Source: CAD feature listing. Evaluate the final solid. Frame: model axes, mm. Face numbers are marked on the shaded views. A direction names the side the tool comes from. Round coordinates to 2 decimals unless told otherwise and drop trailing zeros. Order: outer loops, then holes, each group sorted by start corner. A loop starts at its lowest first (then second) coordinate and runs counter-clockwise, first axis right, second up. Notation, with made-up numbers: M -12.75,17 L -6.75,17 A27 ccw -6.75,51 Z; hole C -12.5,73.25 d9. An arc over 180 degrees is marked long. Use one line per item in the form item = value. Start each with the question number.
Q1. Pull-direction query (X, two-part tool) for the marked faces 4, 5, 6 and 7; classes: pulls with the +X half, pulls with the -X half, needs draft (parallel to the pull), parting line crosses it, or undercut.
Q2. Section A-A (x = 13.5). Return the cut outline in (y, z), plus the area to 3 significant figures.
Q3. Section B-B (y = 2.3). Give the number of separate pieces and of enclosed holes in the cut face, plus the area to 3 significant figures.
Q4. Material intervals for probe 1 along X at (y, z) = (2.5, -6); probe 2 along Z at (x, y) = (52, 0.9); probe 3 along Z at (x, y) = (52, 1.15), sorted ascending.
Q5. Reachability of the marked faces 1, 2 and 3 from +Z, -Z, +X, -X, +Y, -Y: full face, straight path, thin tool, end or side. Return the list, or none.
Q6. Contact query for flat-ended pins moving along their axis: pin 1 (1.5 mm diameter, centred on x = 33.5, y = 4, fed in from -Z); pin 2 (1.5 mm diameter, centred on y = 2, z = -0.5, fed in from +X); pin 3 (3.5 mm diameter, centred on x = 0, z = 0, fed in from -Y); pin 4 (2.5 mm diameter, centred on x = 37, z = 0, fed in from -Y). Output: stop coordinate, or through.
from build123d import *

# Parameters (mm, degrees)
SKETCH1_W           = 10
SKETCH1_H           = 6
BOSS_EXTRUDE1_DEPTH = 5
BOSS_EXTRUDE3_DEPTH = 1
BOSS_EXTRUDE4_DEPTH = 7
SKETCH4_W           = 6
SKETCH4_H           = 5
BOSS_EXTRUDE5_DEPTH = 30
SKETCH5_W           = 14
SKETCH5_H           = 10
BOSS_EXTRUDE6_DEPTH = 5
FILLET17_R          = 5
SKETCH8_W           = 18
SKETCH8_H           = 5
BOSS_EXTRUDE7_DEPTH = 6
FILLET8_R           = 1
CUT_EXTRUDE3_DEPTH  = 15
SKETCH10_R          = 1.6
CUT_EXTRUDE4_DEPTH  = 57.311632901
FILLET11_R          = 3
CUT_EXTRUDE9_DEPTH  = 1
SKETCH14_W          = 6
SKETCH14_H          = 5
CUT_EXTRUDE10_DEPTH = 1


with BuildPart() as part:
    # Sketch1 → Boss-Extrude1 (new body)
    with BuildSketch(Plane(origin=(0, 0, 0), x_dir=(1, 0, 0), z_dir=(0, 1, 0))):
        Rectangle(SKETCH1_W, SKETCH1_H)
    extrude(amount=BOSS_EXTRUDE1_DEPTH)

    # Sketch2 → Boss-Extrude3 (add)
    with BuildSketch(Plane.XY.offset(3)):
        with BuildLine():
            Line((-5, 0), (5, 0))
            ThreePointArc((5, 0), (0, 5), (-5, 0))
        make_face()
    boss_extrude3 = extrude(amount=BOSS_EXTRUDE3_DEPTH)

    # Sketch3 → Boss-Extrude4 (add)
    with BuildSketch(Plane.XY.offset(4)):
        with BuildLine():
            Line((-3.9, 0), (3.9, 0))
            ThreePointArc((3.9, 0), (0, 3.9), (-3.9, 0))
        make_face()
    boss_extrude4 = extrude(amount=BOSS_EXTRUDE4_DEPTH)

    # Mirror1: Boss-Extrude3, Boss-Extrude4 across plane
    add(boss_extrude3.mirror(Plane.XY))
    add(boss_extrude4.mirror(Plane.XY))

    # Sketch4 → Boss-Extrude5 (add)
    with BuildSketch(Plane(origin=(5, 0, 0), x_dir=(0, 0, -1), z_dir=(1, 0, 0))):
        with Locations((0, 2.5)):
            Rectangle(SKETCH4_W, SKETCH4_H)
    extrude(amount=BOSS_EXTRUDE5_DEPTH)

    # Sketch5 → Boss-Extrude6 (add)
    with BuildSketch(Plane(origin=(0, 0, 0), x_dir=(1, 0, 0), z_dir=(0, 1, 0))):
        with Locations((42, 0)):
            Rectangle(SKETCH5_W, SKETCH5_H)
    extrude(amount=BOSS_EXTRUDE6_DEPTH)

    # Fillet17
    fillet17_edges = [part.edges().sort_by_distance(p)[0] for p in [
        (-5, 5, 0),
    ]]
    fillet(fillet17_edges, radius=FILLET17_R - 0.0001)  # a hair under: the kernel refuses the full size

    # Sketch8 → Boss-Extrude7 (add)
    with BuildSketch(Plane(origin=(49, 0, 0), x_dir=(0, 0, -1), z_dir=(1, 0, 0))):
        with Locations((0, 2.5)):
            Rectangle(SKETCH8_W, SKETCH8_H)
    extrude(amount=BOSS_EXTRUDE7_DEPTH)

    # Fillet8
    fillet8_edges = [part.edges().sort_by_distance(p)[0] for p in [
        (49, 2.5, 5),
        (35, 2.5, 5),
        (35, 2.5, 3),
        (35, 2.5, -3),
        (35, 2.5, -5),
        (49, 2.5, -5),
    ]]
    fillet(fillet8_edges, radius=FILLET8_R - 0.0001)  # a hair under: the kernel refuses the full size

    # Sketch9 → Cut-Extrude3 (cut)
    with BuildSketch(Plane(origin=(55, 0, 0), x_dir=(0, 0, -1), z_dir=(1, 0, 0))):
        with BuildLine():
            Line((-3, 0), (3, 0))
            ThreePointArc((3, 0), (0, 3), (-3, 0))
        make_face()
    extrude(amount=-CUT_EXTRUDE3_DEPTH, mode=Mode.SUBTRACT)

    # Sketch10 → Cut-Extrude4 (cut, through all)
    with BuildSketch(Plane.XZ):
        with Locations(Location((52, 6, 0), (0, 0, 270))):
            Circle(SKETCH10_R)
        with Locations(Location((52, -6, 0), (0, 0, 270))):
            Circle(SKETCH10_R)
        with Locations(Location((37, 0, 0), (0, 0, 270))):
            Circle(SKETCH10_R)
        with Locations(Location((0, 0, 0), (0, 0, 270))):
            Circle(SKETCH10_R)
    extrude(amount=-CUT_EXTRUDE4_DEPTH, mode=Mode.SUBTRACT)

    # Fillet11
    fillet11_edges = [part.edges().sort_by_distance(p)[0] for p in [
        (49, 2.5, -9),
        (55, 2.5, -9),
        (49, 2.5, 9),
        (55, 2.5, 9),
    ]]
    fillet(fillet11_edges, radius=FILLET11_R - 0.0001)  # a hair under: the kernel refuses the full size

    # Sketch13 → Cut-Extrude9 (cut)
    with BuildSketch(Plane(origin=(0, 5, 0), x_dir=(1, 0, 0), z_dir=(0, 1, 0))):
        Polygon((55.290896534, -6), (53.645448267, -3.15), (50.354551733, -3.15), (48.709103466, -6), (50.354551733, -8.85), (53.645448267, -8.85), align=None)
        Polygon((55.290896534, 6), (53.645448267, 8.85), (50.354551733, 8.85), (48.709103466, 6), (50.354551733, 3.15), (53.645448267, 3.15), align=None)
        Polygon((39.85, -1.645448267), (39.85, 1.645448267), (37, 3.290896534), (34.15, 1.645448267), (34.15, -1.645448267), (37, -3.290896534), align=None)
        Polygon((0, -3.290896534), (2.85, -1.645448267), (2.85, 1.645448267), (0, 3.290896534), (-2.85, 1.645448267), (-2.85, -1.645448267), align=None)
    extrude(amount=-CUT_EXTRUDE9_DEPTH, mode=Mode.SUBTRACT)

    # Sketch14 → Cut-Extrude10 (cut)
    with BuildSketch(Plane(origin=(0, 5, 0), x_dir=(1, 0, 0), z_dir=(0, 1, 0))):
        with Locations((52, -7.996152423)):
            Rectangle(SKETCH14_W, SKETCH14_H)
        with Locations((52, 7.996152423)):
            Rectangle(SKETCH14_W, SKETCH14_H)
    extrude(amount=-CUT_EXTRUDE10_DEPTH, mode=Mode.SUBTRACT)


solid = part.part
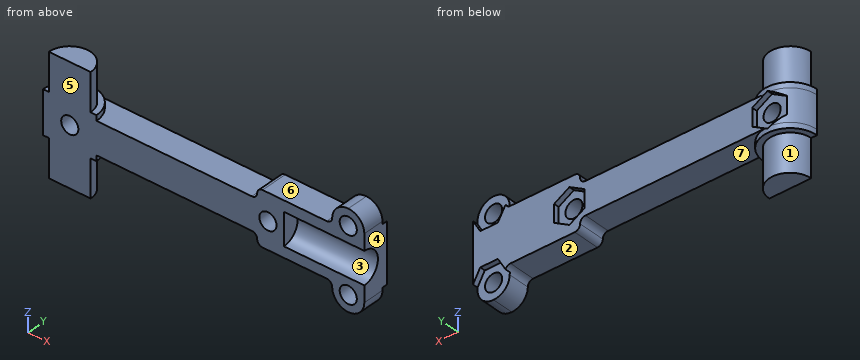
Results list:
q1.face_4 = pulls with the +X half
q1.face_5 = needs draft
q1.face_6 = undercut
q1.face_7 = undercut
q2.outline = M 0,-3 L 5,-3 L 5,3 L 0,3 Z
q2.area = 30.0 mm2
q3.separate_pieces = 1
q3.enclosed_holes = 4
q3.area = 493 mm2
q4.probe_1 = -2.99 to 2.99, 49 to 50.4, 53.6 to 55
q4.probe_2 = -9 to -7.6, -4.4 to -2.86, 2.86 to 4.4, 7.6 to 9
q4.probe_3 = -9 to -7.6, -4.4 to -2.77, 2.77 to 4.4, 7.6 to 9
q5.face_1 = -Z, +Y
q5.face_2 = -Z, +Y, -Y
q5.face_3 = +X, -Y
q6.pin_1 = -3.03
q6.pin_2 = 40
q6.pin_3 = 0
q6.pin_4 = through
